Read the model definition and answer for the solid it produces. Units are mm, in the model's axes. Give positions to 0.01 mm unless a question says otherwise; leave off trailing zeros. Write each loop counter-clockwise with the first axis right and the second up, starting at its lowest first coordinate (ties: lowest second). Pieces come first, ordered by that corner, then holes. Notation, with made-up numbers: M -5,34 L 25,34 A12 cw 25,50 Z; hole C 15,34 d11. An arc over 180 degrees is marked long. Answer as CSV lines item,"result". Start each with the question number.
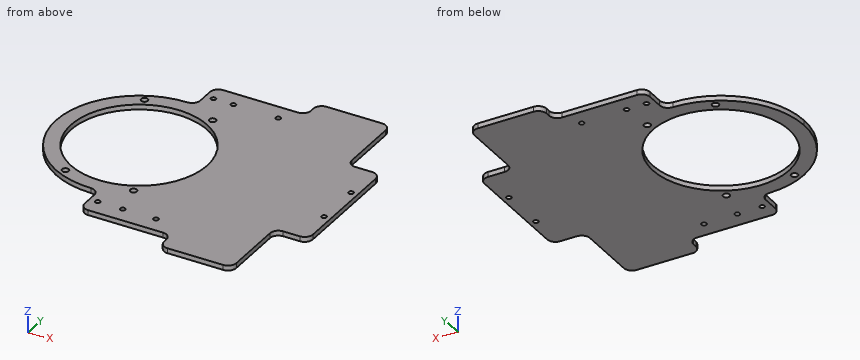
```python
from build123d import *

# Parameters (mm, degrees)
SKETCH_1_W          = 110
SKETCH_1_H          = 100
SKETCH_1_W_2        = 55
SKETCH_1_H_2        = 20
EXTRUDE_1_DEPTH     = 3
FILLET_1_R          = 50
SKETCH_2_R          = 41
CUT_EXTRUDE_1_DEPTH = 10
FILLET_4_R          = 5
SKETCH_3_R          = 1.5
SKETCH_3_R_2        = 2
CUT_EXTRUDE_2_DEPTH = 10
SKETCH_4_W          = 20
SKETCH_4_H          = 45
CUT_EXTRUDE_3_DEPTH = 10
FILLET_5_R          = 5


with BuildPart() as part:
    # 草图1 → 凸台-拉伸1 (new body)
    with BuildSketch(Plane.XY):
        Rectangle(SKETCH_1_W, SKETCH_1_H)
        Polygon((55, 70), (55, 50), (55, -50), (55, -70), (55, -82.5), (118.5, -82.5), (118.5, 82.5), (55, 82.5), align=None)
        with Locations((27.5, 60)):
            Rectangle(SKETCH_1_W_2, SKETCH_1_H_2)
        with Locations((27.5, -60)):
            Rectangle(SKETCH_1_W_2, SKETCH_1_H_2)
    extrude(amount=EXTRUDE_1_DEPTH)

    # 圆角1
    fillet_1_edges = [part.edges().sort_by_distance(p)[0] for p in [
        (-55, -50, 1.5),
        (-55, 50, 1.5),
    ]]
    fillet(fillet_1_edges, radius=FILLET_1_R - 0.0001)  # a hair under: the kernel refuses the full size

    # 草图2 → 切除-拉伸1 (cut)
    with BuildSketch(Plane.XY.offset(3)):
        with Locations((-5, 0)):
            Circle(SKETCH_2_R)
    extrude(amount=-CUT_EXTRUDE_1_DEPTH, mode=Mode.SUBTRACT)

    # 圆角4
    fillet_4_edges = [part.edges().sort_by_distance(p)[0] for p in [
        (0, -70, 1.5),
        (0, -50, 1.5),
        (0, 50, 1.5),
        (0, 70, 1.5),
        (55, 70, 1.5),
        (55, -70, 1.5),
    ]]
    fillet(fillet_4_edges, radius=FILLET_4_R)

    # 草图3 → 切除-拉伸2 (cut)
    with BuildSketch(Plane.XY.offset(3)):
        with Locations((114.5, 14)):
            Circle(SKETCH_3_R)
        with Locations((114.5, -14)):
            Circle(SKETCH_3_R)
        with Locations((-25.5, 41)):
            Circle(SKETCH_3_R_2)
        with Locations((15.5, 41)):
            Circle(SKETCH_3_R_2)
        with Locations((15.5, -41)):
            Circle(SKETCH_3_R_2)
        with Locations((-25.5, -41)):
            Circle(SKETCH_3_R_2)
        with Locations((5, -60)):
            Circle(SKETCH_3_R)
        with Locations((20, -60)):
            Circle(SKETCH_3_R)
        with Locations((40, -60)):
            Circle(SKETCH_3_R)
        with Locations((5, 60)):
            Circle(SKETCH_3_R)
        with Locations((17, 60)):
            Circle(SKETCH_3_R)
        with Locations((44, 60)):
            Circle(SKETCH_3_R)
    extrude(amount=-CUT_EXTRUDE_2_DEPTH, mode=Mode.SUBTRACT)

    # 草图4 → 切除-拉伸3 (cut)
    with BuildSketch(Plane.XY.offset(3)):
        with Locations((108.5, 60)):
            Rectangle(SKETCH_4_W, SKETCH_4_H)
        with Locations((108.5, -60)):
            Rectangle(SKETCH_4_W, SKETCH_4_H)
    extrude(amount=-CUT_EXTRUDE_3_DEPTH, mode=Mode.SUBTRACT)

    # 圆角5
    fillet_5_edges = [part.edges().sort_by_distance(p)[0] for p in [
        (98.5, 82.5, 1.5),
        (118.5, 37.5, 1.5),
        (98.5, 37.5, 1.5),
        (98.5, -82.5, 1.5),
        (98.5, -37.5, 1.5),
        (118.5, -37.5, 1.5),
        (55, 82.5, 1.5),
        (55, -82.5, 1.5),
    ]]
    fillet(fillet_5_edges, radius=FILLET_5_R)


solid = part.part
```
1. Find section A-A on x = -19.5. Determine the outline of the cut face in (y, z).
2. Find the intervals of material crossed by line 1 (Y direction, x = -5.5, z = 1.2); line 2 (Y direction, x = 40, z = 2); line 3 (Y direction, x = 17, z = 2.1), in increasing order. Write a range as [from, to].
3. Find section C-C on z = 1.4. State how many separate pieces and enclosed holes the cut face has, then the cut area to 3 significant figures.
4. Find section B-B on y = 2. Determine the outline of the cut face in (x, z), then the cut area to 3 significant figures.
5. Given pin 1 (0.9 mm diameter, centred on x = 107, z = 2, fed in from +Y); pin 2 (0.9 mm diameter, centred on x = 106.5, z = 2, fed in from -Y); pin 3 (1 mm diameter, centred on x = 43.5, z = 2.5, fed in from +Y), each flat-ended and moving along its own axis, determine where each tip first touches the part or whether it passes through.
Computed:
1,outline,"M -47.85,0 L -38.35,0 L -38.35,3 L -47.85,3 Z; M 38.35,0 L 47.85,0 L 47.85,3 L 38.35,3 Z"
2,line 1,"y = [-50, -41], [41, 50]"
2,line 2,"y = [-70, -61.5], [-58.5, 70]"
2,line 3,"y = [-70, -42.32], [-39.68, -34.6], [34.6, 39.68], [42.32, 58.5], [61.5, 70]"
3,separate pieces,"1"
3,enclosed holes,"13"
3,area,"15,400 mm^2"
4,outline,"M -54.96,0 L -45.95,0 L -45.95,3 L -54.96,3 Z; M 35.95,0 L 118.5,0 L 118.5,3 L 35.95,3 Z"
4,area,"275 mm^2"
5,pin 1,"stops at y = 37.5"
5,pin 2,"stops at y = -37.5"
5,pin 3,"stops at y = 70"
